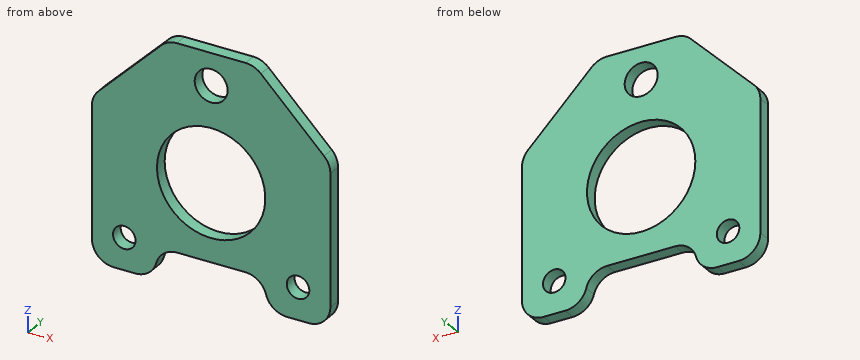
Autodesk Inventor part; units mm, degrees
ref_plane "YZ Plane" through (0, 0, 0) normal (1, 0, 0) x (0, 1, 0)
ref_plane "XZ Plane" through (0, 0, 0) normal (0, 1, 0) x (-1, 0, 0)
ref_plane "XY Plane" through (0, 0, 0) normal (0, 0, 1) x (1, 0, 0)
sketch "Sketch1" plane through (0, 0, 0) normal (0, 1, 0) x (-1, 0, 0)
  line L0 (0, 0) -> (55, 0)
  line L1 (55, 0) -> (55, -55)
  line L2 (55, -55) -> (0, -55)
  line L3 (0, -55) -> (0, 0)
  line L4 (47.55, -7.45) -> (7.45, -7.45) construction
  line L5 (7.45, -7.45) -> (7.45, -47.55) construction
  line L6 (7.45, -47.55) -> (47.55, -47.55) construction
  line L7 (47.55, -47.55) -> (47.55, -7.45) construction
  circle A0 centre (47.55, -47.55) radius 2.6
  circle A1 centre (7.45, -47.55) radius 2.6
  circle A2 centre (27.5, -7.45) radius 3.8
  line L8 (0, -17.5) -> (17.5, 0)
  line L9 (37.5, 0) -> (55, -17.5)
  line L10 (17.5, -55) -> (37.5, -55)
  line L11 (15, -55) -> (40, -55)
  line L12 (40, -55) -> (40, -47.55)
  line L13 (40, -47.55) -> (15, -47.55)
  line L14 (15, -47.55) -> (15, -55)
  circle A3 centre (27.5, -29.55) radius 12.5
  dimension "d0" = 55
  dimension "d1" = 55
  dimension "d2" = 40.1
  dimension "d3" = 40.1
  dimension "d6" = 5.2
  dimension "d7" = 5.2
  dimension "d8" = 7.45
  dimension "d9" = 7.45
  dimension "d14" = 7.6
  dimension "d55" = 20
  dimension "d56" = 10
  dimension "d87" = 15
  dimension "d88" = 15
  dimension "d89" = 25
  dimension "d90" = 18
  dimension "d91" = 20.05
extrude "Extrusion1" add sketch "Sketch1" along normal blind 3 contours L0 L9 L1 L2 L12 L13 L14 L3 L8
fillet "Fillet1" radius 5 10 edges at (-55, 1.5, -55) (0, 1.5, -55) (-55, 1.5, -17.5) (-37.5, 1.5, 0) (-17.5, 1.5, 0) (0, 1.5, -17.5) (-15, 1.5, -55) (-40, 1.5, -55) (-15, 1.5, -47.55) (-40, 1.5, -47.55)
equation "\"d1\" = d0"
equation "\"d3\" = d2"
equation "\"d8\" = -0.5 * d2 + 0.5 * d0"
equation "\"d9\" = -0.5 * d3 + 0.5 * d1"
equation "\"d88\" = d87"
equation "\"d91\" = 0.5 * d2"
properties part number "Gantry Plate" material "PC/ABS Plastic"
Read the model definition and answer for the solid it produces. Units are mm, in the model's axes. Give positions to 0.01 mm unless a question says otherwise; leave off trailing zeros. Write each loop counter-clockwise with the first axis right and the second up, starting at its lowest first coordinate (ties: lowest second). Pieces come first, ordered by that corner, then holes. Notation, with made-up numbers: (64, 59.5) - (83, 59.5) arc R22 ccw to (83, 85.5) - close; hole circle Ø4 at (0.5, 0.5). An arc over 180 degrees is marked (long way). Return JSON: item names as keys, results as strings.
Q1. A cutting plane is placed at D-D, the plane z = -46.5. Determine the outline of the cut face in (x, y).
Reply:
{"outline": "(-55, 0) - (-49.93, 0) - (-49.93, 3) - (-55, 3) - close; (-45.17, 0) - (-9.83, 0) - (-9.83, 3) - (-45.17, 3) - close; (-5.07, 0) - (0, 0) - (0, 3) - (-5.07, 3) - close"}
Q2. A cutting plane is placed at A-A, the plane x = -27.5. Determine the outline of the cut face in (y, z).
Reply:
{"outline": "(0, -47.55) - (3, -47.55) - (3, -42.05) - (0, -42.05) - close; (0, -17.05) - (3, -17.05) - (3, -11.25) - (0, -11.25) - close; (0, -3.65) - (3, -3.65) - (3, 0) - (0, 0) - close"}
Q3. Given P1, Ø1.5, axis at x = -38.5, y = 1, coming from the +Z side; P2, Ø1, axis at x = -46.5, y = 1.5, coming from the +Z side, each flat-ended and moving along its own axis, determine where each tip first touches the part or whether it passes through.
Reply:
{"P1": "z = -0.57", "P2": "z = -8.5"}
Q4. A cutting plane is placed at C-C, the plane x = -7.45. Determine the outline of the cut face in (y, z).
Reply:
{"outline": "(0, -55) - (3, -55) - (3, -50.15) - (0, -50.15) - close; (0, -44.95) - (3, -44.95) - (3, -10.05) - (0, -10.05) - close"}
Q5. Consider line 1 along Z through (x, y) = (-27.5, 2.4); line 2 along Z through (x, y) = (-7.45, 1.3); line 3 along X through (y, z) = (0.45, -8). Determine where each line is inside the solid, lowest interval first. Write a range as [from, to].
Reply:
{"line 1": "[-47.55, -42.05], [-17.05, -11.25], [-3.65, 0]", "line 2": "[-55, -50.15], [-44.95, -10.05]", "line 3": "[-45.5, -31.26], [-23.74, -9.5]"}
Q6. A cutting plane is placed at B-B, the plane z = -29.55. Determine the outline of the cut face in (x, y), and give its area (3 significant figures).
Reply:
{"outline": "(-55, 0) - (-40, 0) - (-40, 3) - (-55, 3) - close; (-15, 0) - (0, 0) - (0, 3) - (-15, 3) - close", "area": "90.0 mm²"}
